```python
from build123d import *

# Parameters (mm, degrees)
BOSS_EXTRUDE1_DEPTH = 6
SKETCH2_R           = 9.15
SKETCH2_R_2         = 8.15
BOSS_EXTRUDE2_DEPTH = 7.4
CUT_EXTRUDE1_DEPTH  = 3
SKETCH4_R           = 1.75
CUT_EXTRUDE2_DEPTH  = 45.359440934
SKETCH5_W           = 3
SKETCH5_H           = 5.3
SKETCH5_W_2         = 6.7
SKETCH5_H_2         = 6.7
CUT_EXTRUDE3_DEPTH  = 3


with BuildPart() as part:
    # Sketch1 → Boss-Extrude1 (new body)
    with BuildSketch(Plane(origin=(0, 0, 0), x_dir=(1, 0, 0), z_dir=(0, 1, 0))):
        with BuildLine():
            Line((-31.2, 10.6), (31.2, 10.6))
            ThreePointArc((31.2, 10.6), (41.8, 0), (31.2, -10.6))
            Line((31.2, -10.6), (-31.2, -10.6))
            ThreePointArc((-31.2, -10.6), (-41.8, 0), (-31.2, 10.6))
        make_face()
    extrude(amount=BOSS_EXTRUDE1_DEPTH)

    # Sketch2 → Boss-Extrude2 (add)
    # profile 1 of 2: a face of its own
    with BuildSketch(Plane(origin=(0, 6, 0), x_dir=(1, 0, 0), z_dir=(0, 1, 0))):
        with Locations(Location((-21.65, 0, 0), (0, 0, 270))):
            Circle(SKETCH2_R)
        with Locations(Location((-21.65, 0, 0), (0, 0, 270))):
            Circle(SKETCH2_R_2, mode=Mode.SUBTRACT)
    # profile 2 of 2: a face of its own
    with BuildSketch(Plane(origin=(0, 6, 0), x_dir=(1, 0, 0), z_dir=(0, 1, 0))):
        with Locations(Location((-3.2, 0, 0), (0, 0, 270))):
            Circle(SKETCH2_R)
        with Locations(Location((-3.2, 0, 0), (0, 0, 270))):
            Circle(SKETCH2_R_2, mode=Mode.SUBTRACT)
    extrude(amount=BOSS_EXTRUDE2_DEPTH)

    # Sketch3 → Cut-Extrude1 (cut)
    with BuildSketch(Plane(origin=(0, 6, 0), x_dir=(1, 0, 0), z_dir=(0, 1, 0))):
        Polygon((-37.25, -3.233161507), (-34.45, -1.616580754), (-34.45, 1.616580754), (-37.25, 3.233161507), (-40.05, 1.616580754), (-40.05, -1.616580754), align=None)
        Polygon((37.25, -3.233161507), (40.05, -1.616580754), (40.05, 1.616580754), (37.25, 3.233161507), (34.45, 1.616580754), (34.45, -1.616580754), align=None)
    extrude(amount=-CUT_EXTRUDE1_DEPTH, mode=Mode.SUBTRACT)

    # Sketch4 → Cut-Extrude2 (cut, through all)
    with BuildSketch(Plane(origin=(0, 3, 0), x_dir=(1, 0, 0), z_dir=(0, 1, 0))):
        with Locations(Location((-37.25, 0, 0), (0, 0, 270))):
            Circle(SKETCH4_R)
        with Locations(Location((37.25, 0, 0), (0, 0, 270))):
            Circle(SKETCH4_R)
    extrude(amount=-CUT_EXTRUDE2_DEPTH, mode=Mode.SUBTRACT)

    # Sketch5 → Cut-Extrude3 (cut)
    with BuildSketch(Plane(origin=(0, 6, 0), x_dir=(1, 0, 0), z_dir=(0, 1, 0))):
        with Locations((24.75, -2.75)):
            Rectangle(SKETCH5_W, SKETCH5_H)
        with Locations((15.7, 0.75)):
            Rectangle(SKETCH5_W_2, SKETCH5_H_2)
    extrude(amount=-CUT_EXTRUDE3_DEPTH, mode=Mode.SUBTRACT)


solid = part.part
```
For this review, take the finished solid that the model builds, in its own axes (mm). A direction names the side the tool comes from. Round coordinates to 2 decimals unless told otherwise and drop trailing zeros. Write each loop counter-clockwise with the first axis right and the second up, starting at its lowest first coordinate (ties: lowest second). Pieces come first, ordered by that corner, then holes. Notation, with made-up numbers: (63, 80.25) -> (97, 80.25) arc R25 ccw to (97, 97.25) -> close; hole circle Ø3 at (20, 49). An arc over 180 degrees is marked (long way). Use one line per item in the form item = value.
1) To check wall thickness, follow L1, parallel to X at y = 1.6, z = 0; L2, parallel to X at y = 10.25, z = 0; L3, parallel to X at y = 11.25, z = 6.5. State the ranges of each line that lie inside material, in increasing order. Write a range as from..to.
Found:
L1 = -41.8..-39, -35.5..35.5, 39..41.8
L2 = -30.8..-29.8, -13.5..-12.5, -12.35..-11.35, 4.95..5.95
L3 = -28.09..-26.57, -16.73..-15.21, -9.64..-8.12, 1.72..3.24
2) Take a section at B-B, the plane x = -3.2. Write out the cut boundary in (y, z).
Found:
outline = (0, -10.6) -> (6, -10.6) -> (6, -9.15) -> (13.4, -9.15) -> (13.4, -8.15) -> (6, -8.15) -> (6, 8.15) -> (13.4, 8.15) -> (13.4, 9.15) -> (6, 9.15) -> (6, 10.6) -> (0, 10.6) -> close
3) Take a section at C-C, the plane y = 12.25. Write out the cut boundary in (x, z).
Found:
outline = circle Ø18.3 at (-21.65, 0); circle Ø18.3 at (-3.2, 0); hole circle Ø16.3 at (-21.65, 0); hole circle Ø16.3 at (-3.2, 0)
4) Take a section at D-D, the plane z = 4.25. Write out the cut boundary in (x, y), and give its area (3 significant figures).
Found:
outline = (-40.91, 0) -> (40.91, 0) -> (40.91, 6) -> (26.25, 6) -> (26.25, 3) -> (23.25, 3) -> (23.25, 6) -> (4.9, 6) -> (4.9, 13.4) -> (3.75, 13.4) -> (3.75, 6) -> (-10.15, 6) -> (-10.15, 13.4) -> (-11.3, 13.4) -> (-11.3, 6) -> (-13.55, 6) -> (-13.55, 13.4) -> (-14.7, 13.4) -> (-14.7, 6) -> (-28.6, 6) -> (-28.6, 13.4) -> (-29.75, 13.4) -> (-29.75, 6) -> (-40.91, 6) -> close
area = 516 mm2
5) Tool access review of faces 1 (the cylindrical face through (-39, 2, 0)), 2 (the flat face through (-38.63, 4.521, -2.436)): name each direction out of +Z, -Z, +X, -X, +Y, -Y from which nothing blocks a thin tool from reaching the whole face with its end or side.
Found:
face_1 = +Y, -Y
face_2 = +Y
6) Mouldability with a two-part tool opening along Z and no side actions: class faces 3 (the flat face through (1, 0, 0)), 4 (the cylindrical face through (41.8, 3, -0.2)), 5 (the flat face through (-40.05, 5, 0)) as +Z half, -Z half, draft (parallel to the pull), parting line (faces both ways), or undercut.
Found:
face_3 = draft
face_4 = parting line
face_5 = undercut
7) Take a section at A-A, the plane y = 5. Write out the cut boundary in (x, z).
Found:
outline = (-31.2, -10.6) -> (31.2, -10.6) arc R10.6 ccw to (31.2, 10.6) -> (-31.2, 10.6) arc R10.6 ccw to start; hole (-40.05, -1.62) -> (-37.25, -3.23) -> (-34.45, -1.62) -> (-34.45, 1.62) -> (-37.25, 3.23) -> (-40.05, 1.62) -> close; hole (12.35, -4.1) -> (19.05, -4.1) -> (19.05, 2.6) -> (12.35, 2.6) -> close; hole (23.25, 0.1) -> (26.25, 0.1) -> (26.25, 5.4) -> (23.25, 5.4) -> close; hole (34.45, -1.62) -> (37.25, -3.23) -> (40.05, -1.62) -> (40.05, 1.62) -> (37.25, 3.23) -> (34.45, 1.62) -> close
8) Clearance check with flat-ended pins moving along their axes: pin 1 (1.5 mm diameter, centred on y = 5, z = -1, fed in from +X); pin 2 (8 mm diameter, centred on x = -28, y = 12, fed in from +Z); pin 3 (4 mm diameter, centred on x = 32, z = -6.5, fed in from +Y). State where each tip first meets the part, or that it passes through.
Found:
pin_1 = 41.8
pin_2 = 8.84
pin_3 = 6
